```python
from build123d import *

# Parameters (mm, degrees)
SKETCH1_W           = 88.9
SKETCH1_H           = 38.1
BOSS_EXTRUDE1_DEPTH = 546.1
FILLET1_R           = 2
SKETCH2_R           = 6.35
CUT_EXTRUDE1_DEPTH  = 550.229116581


with BuildPart() as part:
    # Sketch1 → Boss-Extrude1 (new body)
    with BuildSketch(Plane(origin=(0, 0, 0), x_dir=(0, 0, -1), z_dir=(1, 0, 0))):
        Rectangle(SKETCH1_W, SKETCH1_H)
    extrude(amount=BOSS_EXTRUDE1_DEPTH)

    # Fillet1
    fillet1_edges = [part.edges().sort_by_distance(p)[0] for p in [
        (273.05, -19.05, -44.45),
        (273.05, -19.05, 44.45),
        (273.05, 19.05, 44.45),
        (273.05, 19.05, -44.45),
    ]]
    fillet(fillet1_edges, radius=FILLET1_R)

    # Sketch2 → Cut-Extrude1 (cut, through all)
    with BuildSketch(Plane(origin=(0, 19.05, 0), x_dir=(1, 0, 0), z_dir=(0, 1, 0))):
        with Locations(Location((38.1, 0, 0), (0, 0, 270))):
            Circle(SKETCH2_R)
        with Locations(Location((508, 0, 0), (0, 0, 270))):
            Circle(SKETCH2_R)
    extrude(amount=-CUT_EXTRUDE1_DEPTH, mode=Mode.SUBTRACT)


solid = part.part
```
Verification items for the finished model (mm, model axes). Round coordinates to 2 decimals unless told otherwise and drop trailing zeros. Write each loop counter-clockwise with the first axis right and the second up, starting at its lowest first coordinate (ties: lowest second). Pieces come first, ordered by that corner, then holes. Notation, with made-up numbers: (42.25, 9.5) -> (69.25, 9.5) arc R8 cw to (69.25, 23.5) -> close; hole circle Ø5 at (-20.75, -10). An arc over 180 degrees is marked (long way). Write each question's results on one line, items separated by ' | '. Start each with the question number.
1. Cross-section at A-A (x = 38.1). Enter the section's corners in (y, z).
2. Cross-section at B-B (z = 0). Enter the section's corners in (x, y), then the cut area to 3 significant figures.
3. Material ranges on probe 1 along X at (y, z) = (-0.5, 0); probe 2 along Z at (x, y) = (508, -7); probe 3 along X at (y, z) = (17.5, -5.5), recorded low to high. Write a range as from..to.
4. Draft check along Z on faces 1 (the flat face through (546.1, 0, 1)), 2 (the cylindrical face through (31.9, 0.27, -1.38)), 3 (the flat face through (269, 0, -44.45)). Enter one of: +Z half, -Z half, draft (parallel to the pull), parting line (faces both ways), or undercut.
Solutions:
1) outline: (-19.05, -42.45) arc R2 ccw to (-17.05, -44.45) -> (17.05, -44.45) arc R2 ccw to (19.05, -42.45) -> (19.05, -6.35) -> (-19.05, -6.35) -> close; (-19.05, 6.35) -> (19.05, 6.35) -> (19.05, 42.45) arc R2 ccw to (17.05, 44.45) -> (-17.05, 44.45) arc R2 ccw to (-19.05, 42.45) -> close
2) outline: (0, -19.05) -> (31.75, -19.05) -> (31.75, 19.05) -> (0, 19.05) -> close; (44.45, -19.05) -> (501.65, -19.05) -> (501.65, 19.05) -> (44.45, 19.05) -> close; (514.35, -19.05) -> (546.1, -19.05) -> (546.1, 19.05) -> (514.35, 19.05) -> close | area: 19,800 mm2
3) probe 1: x = 0..31.75, 44.45..501.65, 514.35..546.1 | probe 2: z = -44.45..-6.35, 6.35..44.45 | probe 3: x = 0..34.93, 41.27..504.83, 511.17..546.1
4) face 1: draft | face 2: undercut | face 3: -Z half
